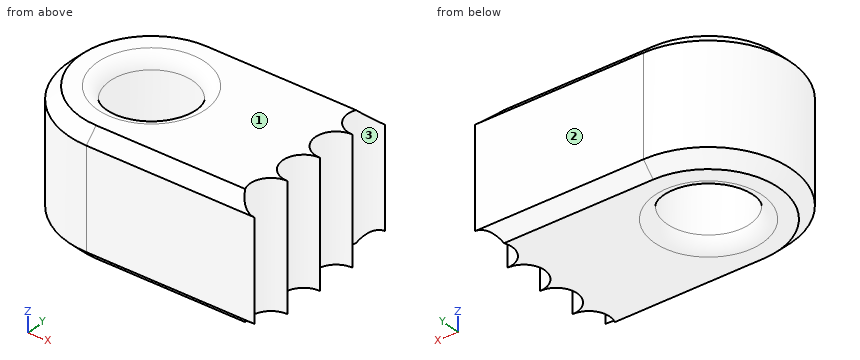
```python
from build123d import *

# Parameters (mm, degrees)
F0_R     = 10
F1_DEPTH = 15
F2_R     = 3
F3_R     = 3
F4_SIZE  = 3
F5_SIZE  = 3


with BuildPart() as f1:
    # F0 (on Top) → F1 (new body, symmetric)
    with BuildSketch(Plane.XY):
        with BuildLine():
            Line((20.557612, 20), (-19.442388, 20))
            ThreePointArc((-19.442388, 20), (-39.442388, 0), (-19.442388, -20))
            Line((-19.442388, -20), (20.557612, -20))
            ThreePointArc((20.557612, -20), (15.557612, -15), (20.557612, -10))
            ThreePointArc((20.557612, -10), (15.557612, -5), (20.557612, 0))
            ThreePointArc((20.557612, 0), (15.557612, 5), (20.557612, 10))
            ThreePointArc((20.557612, 10), (15.557612, 15), (20.557612, 20))
        make_face()
        with Locations((-19.442388, 0)):
            Circle(F0_R, mode=Mode.SUBTRACT)
    extrude(amount=F1_DEPTH, both=True)

    # F2
    f2_edges = [f1.edges().sort_by_distance(p)[0] for p in [
        (-29.442388, 0, 15),
    ]]
    fillet(f2_edges, radius=F2_R)

    # F3
    f3_edges = [f1.edges().sort_by_distance(p)[0] for p in [
        (-29.442388, 0, -15),
    ]]
    fillet(f3_edges, radius=F3_R)

    # F4
    f4_edges = [f1.edges().sort_by_distance(p)[0] for p in [
        (0.557612, 20, 15),
        (-39.442388, 0, 15),
        (0.557612, -20, 15),
    ]]
    chamfer(f4_edges, length=F4_SIZE)

    # F5
    f5_edges = [f1.edges().sort_by_distance(p)[0] for p in [
        (0.557612, -20, -15),
        (-39.442388, 0, -15),
        (0.557612, 20, -15),
    ]]
    chamfer(f5_edges, length=F5_SIZE)


solid = f1.part
```
CAD build for the part. Positions are in the model's coordinates, mm. Face numbers are marked on the shaded views. Coordinates: 2 decimals unless noted, no trailing zeros. Order: outer loops, then holes, each group sorted by start corner. A loop starts at its lowest first (then second) coordinate and runs counter-clockwise, first axis right, second up. Notation, with made-up numbers: (44.5, 9.25) - (85.5, 9.25) arc R11 cw to (85.5, 17.25) - close; hole circle Ø5 at (61, 60.5). An arc over 180 degrees is marked (long way). Use a Markdown table: item, result. Add a question column.
(1) Flat gauge pins, fed straight in: pin 1 (3 mm diameter, centred on y = -3.5, z = 3, fed in from +X); pin 2 (23 mm diameter, centred on x = -19.44, y = 0, fed in from -Z). Where does each tip first touch, or does it go through?
(2) Saw through at B-B (x = -1.5). Give the cut face in (y, z), then the cut area to 3 significant figures.
(3) Drill centre lines: line 1 along Y through (x, z) = (16, -13.25); line 2 along X through (y, z) = (6, 7.75); line 3 along Y through (x, z) = (-24, -12). Where is each one in solid material? Low to high. Write a range as [from, to].
(4) Pull direction Y, two halves, no side cores. Call the marked faces 1, 2 and 3: +Y half, -Y half, draft (parallel to the pull), parting line (faces both ways), or undercut.
(5) Saw through at A-A (z = -8.5). Give the cut face in (x, y).
Solved:
| question | item | result |
|---|---|---|
| 1 | pin 1 | stops at x = 16.56 |
| 1 | pin 2 | stops at z = -14.6 |
| 2 | outline | (-20, -12) - (-17, -15) - (17, -15) - (20, -12) - (20, 12) - (17, 15) - (-17, 15) - (-20, 12) - close |
| 2 | area | 1,180 mm² |
| 3 | line 1 | y = [-18.75, -17.06], [-12.94, -7.06], [-2.94, 2.94], [7.06, 12.94], [17.06, 18.75] |
| 3 | line 2 | x = [-38.52, -27.44], [-11.44, 15.66] |
| 3 | line 3 | y = [-19.47, -8.9], [8.9, 19.47] |
| 4 | face 1 | draft |
| 4 | face 2 | +Y half |
| 4 | face 3 | undercut |
| 5 | outline | (-19.44, -20) - (20.56, -20) arc R5 cw to (20.56, -10) arc R5 cw to (20.56, 0) arc R5 cw to (20.56, 10) arc R5 cw to (20.56, 20) - (-19.44, 20) arc R20 ccw to start; hole circle Ø20 at (-19.44, 0) |
